from build123d import *

# Parameters (mm, degrees)
SKETCH002_R                 = 3
EXTRUDE002_DEPTH            = 6
CYLINDER049_R               = 1.2
CYLINDER049_DEPTH           = 19
CYLINDER014_R               = 2
CYLINDER014_DEPTH           = 5
CYLINDER014_PLACEMENT_ANGLE = 45
CYLINDER015_R               = 2
CYLINDER015_DEPTH           = 5
CYLINDER016_R               = 2
CYLINDER016_DEPTH           = 5
CYLINDER016_PLACEMENT_ANGLE = 135
CYLINDER017_R               = 2
CYLINDER017_DEPTH           = 5
CYLINDER018_R               = 2
CYLINDER018_DEPTH           = 5
CYLINDER018_PLACEMENT_ANGLE = 225
CYLINDER019_R               = 2
CYLINDER019_DEPTH           = 5
CYLINDER020_R               = 2
CYLINDER020_DEPTH           = 5
CYLINDER020_PLACEMENT_ANGLE = 45
CYLINDER013_R               = 2
CYLINDER013_DEPTH           = 5
CYLINDER021_R               = 5
CYLINDER021_DEPTH           = 8
CYLINDER012_R               = 25
CYLINDER012_DEPTH           = 1.5
CUT050_PLACEMENT_ANGLE      = 180


with BuildPart() as extrude002:
    # Sketch002 (on Face25 of Shape005) → Extrude002 (new body)
    with BuildSketch(Plane(origin=(85.664098, -4.553146, 1.091283), x_dir=(-1, 0, 0), z_dir=(0, 0, 1))):
        with Locations((9.450198, -0.000218)):
            Circle(SKETCH002_R)
    extrude(amount=EXTRUDE002_DEPTH)


with BuildPart() as extrude002_1:
    # Extrude002 placement: moved
    add(extrude002.part.moved(Location((-76.21, 4.55, 3))))


with BuildPart() as cylinder049:
    # Cylinder049 → Cylinder049 (new body)
    with BuildSketch(Plane.XY.offset(-1)):
        Circle(CYLINDER049_R)
    extrude(amount=CYLINDER049_DEPTH)


with BuildPart() as cylinder014:
    # cylinder014 → cylinder014 (new body)
    with BuildSketch(Plane.XY):
        Circle(CYLINDER014_R)
    extrude(amount=CYLINDER014_DEPTH)


with BuildPart() as cylinder014_1:
    # cylinder014 placement: moved
    add(cylinder014.part.moved(Location((13.081475, 13.081475, 0))).rotate(Axis((13.081475, 13.081475, 0), (0, 0, 1)), CYLINDER014_PLACEMENT_ANGLE))


with BuildPart() as cylinder015:
    # cylinder015 → cylinder015 (new body)
    with BuildSketch(Plane(origin=(0, 18.5, 0), x_dir=(0, 1, 0), z_dir=(0, 0, 1))):
        Circle(CYLINDER015_R)
    extrude(amount=CYLINDER015_DEPTH)


with BuildPart() as cylinder016:
    # cylinder016 → cylinder016 (new body)
    with BuildSketch(Plane.XY):
        Circle(CYLINDER016_R)
    extrude(amount=CYLINDER016_DEPTH)


with BuildPart() as cylinder016_1:
    # cylinder016 placement: moved
    add(cylinder016.part.moved(Location((-13.081475, 13.081475, 0))).rotate(Axis((-13.081475, 13.081475, 0), (0, 0, 1)), CYLINDER016_PLACEMENT_ANGLE))


with BuildPart() as cylinder017:
    # cylinder017 → cylinder017 (new body)
    with BuildSketch(Plane(origin=(-18.5, 0, 0), x_dir=(-1, 0, 0), z_dir=(0, 0, 1))):
        Circle(CYLINDER017_R)
    extrude(amount=CYLINDER017_DEPTH)


with BuildPart() as cylinder018:
    # cylinder018 → cylinder018 (new body)
    with BuildSketch(Plane.XY):
        Circle(CYLINDER018_R)
    extrude(amount=CYLINDER018_DEPTH)


with BuildPart() as cylinder018_1:
    # cylinder018 placement: moved
    add(cylinder018.part.moved(Location((-13.081475, -13.081475, 0))).rotate(Axis((-13.081475, -13.081475, 0), (0, 0, 1)), CYLINDER018_PLACEMENT_ANGLE))


with BuildPart() as cylinder019:
    # cylinder019 → cylinder019 (new body)
    with BuildSketch(Plane(origin=(0, -18.5, 0), x_dir=(0, -1, 0), z_dir=(0, 0, 1))):
        Circle(CYLINDER019_R)
    extrude(amount=CYLINDER019_DEPTH)


with BuildPart() as cylinder020:
    # cylinder020 → cylinder020 (new body)
    with BuildSketch(Plane.XY):
        Circle(CYLINDER020_R)
    extrude(amount=CYLINDER020_DEPTH)


with BuildPart() as cylinder020_1:
    # cylinder020 placement: moved
    add(cylinder020.part.moved(Location((13.081475, -13.081475, 0))).rotate(Axis((13.081475, -13.081475, 0), (0, 0, -1)), CYLINDER020_PLACEMENT_ANGLE))


with BuildPart() as fusion026:
    # cylinder013 → cylinder013 (new body)
    with BuildSketch(Plane(origin=(18.5, 0, 0), x_dir=(1, 0, 0), z_dir=(0, 0, 1))):
        Circle(CYLINDER013_R)
    extrude(amount=CYLINDER013_DEPTH)

    # Group001: union cylinder014, cylinder015, cylinder016, cylinder017, cylinder018, cylinder019, cylinder020
    add(cylinder014_1.part)
    add(cylinder015.part)
    add(cylinder016_1.part)
    add(cylinder017.part)
    add(cylinder018_1.part)
    add(cylinder019.part)
    add(cylinder020_1.part)


with BuildPart() as fusion026_1:
    # Group001 placement: moved
    add(fusion026.part.moved(Location((0, 0, -1))))

    # Fusion026: union Extrude002, Cylinder049
    add(extrude002_1.part)
    add(cylinder049.part)


with BuildPart() as servo_central_shaft002:
    # cylinder021 → cylinder021 (new body)
    with BuildSketch(Plane.XY):
        Circle(CYLINDER021_R)
    extrude(amount=CYLINDER021_DEPTH)


with BuildPart() as rotor001:
    # cylinder012 → cylinder012 (new body)
    with BuildSketch(Plane.XY):
        Circle(CYLINDER012_R)
    extrude(amount=CYLINDER012_DEPTH)

    # Fusion027: union servo_central_shaft002
    add(servo_central_shaft002.part)

    # Cut050: cut Fusion026
    add(fusion026_1.part, mode=Mode.SUBTRACT)


with BuildPart() as rotor001_1:
    # Cut050 placement: moved
    add(rotor001.part.rotate(Axis((0, 0, 0), (1, 0, 0)), CUT050_PLACEMENT_ANGLE))


solid = rotor001_1.part
The listing builds one solid part. Answer for the finished solid, in the listing's coordinates (mm). A direction names the side the tool comes from. Round coordinates to 2 decimals unless told otherwise and drop trailing zeros. Order: outer loops, then holes, each group sorted by start corner. A loop starts at its lowest first (then second) coordinate and runs counter-clockwise, first axis right, second up. Notation, with made-up numbers: M -33,86 L -12,86 A25 ccw -12,122 Z; hole C 22.5,70.25 d10. An arc over 180 degrees is marked long. Answer in a Markdown table with one row per item. Add a question column.
1) The part is cut by section D-D on x = -8.5. Determine the outline of the cut face in (y, z).
2) Determine the mould class of faces 3 (the face through (-0.1, 3.3, -8)), 4 (the face through (16.9, 1.2, -0.7)), 5 (the face through (-1.08, 4.88, -4.7)) for opening direction X: pulls with the +X half, pulls with the -X half, needs draft (parallel to the pull), parting line crosses it, or undercut.
3) The part is cut by section A-A on y = 18.5. Determine the outline of the cut face in (x, z).
4) The part is cut by section C-C on z = -3. Determine the outline of the cut face in (x, y), plus the area to 3 significant figures.
5) Which of the six approach directions +Z, -Z, +X, -X, +Y, -Y give full straight-line access (tool end or side, diameter ignored) to faces 1 (the face through (-1, -1, -4.091)), 2 (the face through (-11.606, 11.731, -0.74))?
6) Consider line 1 along X through (y, z) = (-14, -0.75); line 2 along Z through (x, y) = (-8.5, -14); line 3 along X through (y, z) = (18.5, -0.75). Determine where each line is inside the solid, lowest interval first. Write a range as from..to.
7) Flat-ended cylindrical pins translate along their axes: pin 1 Ø4.5 at (x, y) = (-13.08, 13.08) entering from -Z; pin 2 Ø2.5 at (x, y) = (13.08, 13.08) entering from +Z; pin 3 Ø2 at (y, z) = (-3.5, -2) entering from +X; pin 4 Ø5 at (x, y) = (0, 0) entering from -Z. Find the tip coordinate at first contact, or state that the pin passes through.
Findings below:
| question | item | result |
|---|---|---|
| 1 | outline | M -23.51,-1.5 L 23.51,-1.5 L 23.51,0 L -23.51,0 Z |
| 2 | face 3 | needs draft |
| 2 | face 4 | undercut |
| 2 | face 5 | parting line crosses it |
| 3 | outline | M -16.82,-1.5 L -2,-1.5 L -2,0 L -16.82,0 Z; M 2,-1.5 L 16.82,-1.5 L 16.82,0 L 2,0 Z |
| 4 | outline | C 0,0 d10; hole C 0,0 d2.4 |
| 4 | area | 74.0 mm² |
| 5 | face 1 | -Z |
| 5 | face 2 | +Z, -Z |
| 6 | line 1 | x = -20.71..-14.86, -11.3..11.3, 14.86..20.71 |
| 6 | line 2 | z = -1.5..0 |
| 6 | line 3 | x = -16.82..-2, 2..16.82 |
| 7 | pin 1 | stops at z = -1.5 |
| 7 | pin 2 | passes through |
| 7 | pin 3 | stops at x = 24.86 |
| 7 | pin 4 | stops at z = -4.09 |
